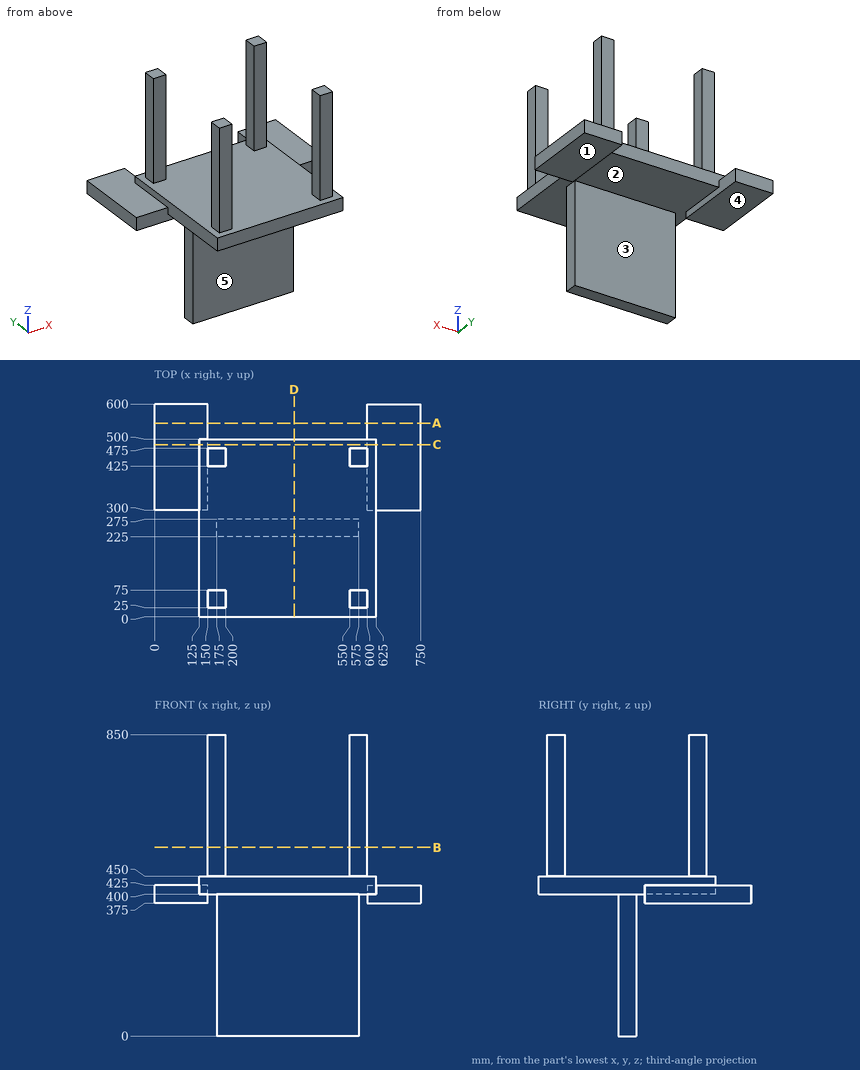
Drawing for the job (mm, zero at the part's lowest x, y, z). A direction names the side the tool comes from. Round coordinates to 2 decimals unless told otherwise and drop trailing zeros. Order: outer loops, then holes, each group sorted by start corner. A loop starts at its lowest first (then second) coordinate and runs counter-clockwise, first axis right, second up. Notation, with made-up numbers: (50, 21.25) -> (61, 21.25) arc R10 cw to (61, 25.25) -> close; hole circle Ø7 at (15, 59.5). An arc over 180 degrees is marked (long way). Write item = value, one per line. Start each with the question number.
(1) Cut at C-C, the plane y = 485.5. List the corners of the cut face in (x, z).
(2) Cut at A-A, the plane y = 546. List the corners of the cut face in (x, z).
(3) Cut at D-D, the plane x = 393. List the corners of the cut face in (y, z), then the cut area to 3 significant figures.
(4) Pin check, flat tips, straight feed: P1, Ø1.5, axis at y = 253.5, z = 341.5, coming from the +X side; P2, Ø25, axis at y = 160.5, z = 431.5, coming from the -X side; P3, Ø1.5, axis at x = 622, y = 282, coming from the +Z side. Stop position of each tip, or through.
(5) Cut at B-B, the plane z = 532. List the corners of the cut face in (x, y), then the cut area to 3 significant figures.
(6) Which spindle directions (+Z, -Z, +X, -X, +Y, -Y) get a long thin tool onto all of the face, cutting with end or side? Do the marked faces 3, 4 and 5. Say none if no direction does.
(7) Probe line 1 (X direction, y = 457, z = 626.5); line 2 (X direction, y = 451, z = 375.5); line 3 (X direction, y = 265, z = 65.5). List the from-to ranges inside material, lowest first. Write a range as [from, to].
(8) Pull direction X, two halves, no side cores. Call the marked faces 1 and 2: released by +X, released by -X, zero draft, split by the parting line, or undercut.
Model answer:
q1.outline = (0, 375) -> (150, 375) -> (150, 400) -> (600, 400) -> (600, 375) -> (750, 375) -> (750, 425) -> (625, 425) -> (625, 450) -> (125, 450) -> (125, 425) -> (0, 425) -> close
q2.outline = (0, 375) -> (150, 375) -> (150, 425) -> (0, 425) -> close; (600, 375) -> (750, 375) -> (750, 425) -> (600, 425) -> close
q3.outline = (0, 400) -> (225, 400) -> (225, 0) -> (275, 0) -> (275, 400) -> (500, 400) -> (500, 450) -> (0, 450) -> close
q3.area = 45,000 mm2
q4.P1 = 575
q4.P2 = 125
q4.P3 = 450
q5.outline = (150, 25) -> (200, 25) -> (200, 75) -> (150, 75) -> close; (150, 425) -> (200, 425) -> (200, 475) -> (150, 475) -> close; (550, 25) -> (600, 25) -> (600, 75) -> (550, 75) -> close; (550, 425) -> (600, 425) -> (600, 475) -> (550, 475) -> close
q5.area = 10,000 mm2
q6.face_3 = -Z, +X, -X, +Y
q6.face_4 = -Z, +X, -X, +Y, -Y
q6.face_5 = -Z, +X, -X, -Y
q7.line_1 = [150, 200], [550, 600]
q7.line_2 = [0, 150], [600, 750]
q7.line_3 = [175, 575]
q8.face_1 = zero draft
q8.face_2 = undercut
